Input: part model. Units: mm. Frame: model coordinates. Round coordinates to 2 decimals unless told otherwise and drop trailing zeros. Loops run counter-clockwise (first coordinate to the right, second up) from the corner with the lowest first, then second, coordinate; pieces in that order, holes last.
1) First-contact query: pin 1 (5 mm diameter, centred on x = -67, z = 0, fed in from -Y); pin 2 (1.5 mm diameter, centred on y = 1, z = 13, fed in from +X). Flat tips, straight axial feed; report the tip coordinate or a pass-through.
2) Section A-A, the plane y = 1.25. State how many separate pieces and enclosed holes the cut face has, and give its area (3 significant figures).
3) Ray query, line 1 along Z through (x, y) = (-250, 2.7); line 2 along Z through (x, y) = (-299.5, 0.8); line 3 along X through (y, z) = (1.5, -8.5). Return the intervals inside material, ascending.
4) Section B-B, the plane z = 26. Return loops of the section in (x, y).
5) Draft query along X for faces 1 (the face through (-187, 0, 0)), 2 (the face through (-294.233, 1.774, -2.999)), 3 (the face through (23.986, 1.774, 24.297)). Return one class per face: pulls with the +X half, pulls with the -X half, needs draft (parallel to the pull), parting line crosses it, or undercut.
Autodesk Inventor part; units mm, degrees
ref_plane "YZ Plane" through (0, 0, 0) normal (1, 0, 0) x (0, 1, 0)
ref_plane "XZ Plane" through (0, 0, 0) normal (0, 1, 0) x (-1, 0, 0)
ref_plane "XY Plane" through (0, 0, 0) normal (0, 0, 1) x (1, 0, 0)
sketch "Sketch1" plane through (0, 0, 0) normal (0, 1, 0) x (-1, 0, 0)
  line L0 (0, 0) -> (-16.25, 0)
  line L1 (0, 0) -> (44.75, 0)
  line L2 (300, 0) -> (330, 0)
  line L3 (330, 30) -> (-30, 30)
  line L4 (-16.25, 15.5) -> (44.75, 15.5)
  line L5 (44.75, 15.5) -> (44.75, 0)
  line L6 (44.75, -15.5) -> (-16.25, -15.5)
  line L7 (-16.25, -15.5) -> (-16.25, 0)
  line L8 (-16.25, 15.5) -> (44.75, -15.5) construction
  line L9 (44.75, 15.5) -> (-16.25, -15.5) construction
  line L10 (-20.25, 8.5) -> (48.75, 8.5) construction
  line L11 (48.75, 8.5) -> (48.75, -8.5) construction
  line L12 (48.75, -8.5) -> (-20.25, -8.5) construction
  line L13 (-20.25, -8.5) -> (-20.25, 8.5) construction
  line L14 (-20.25, 8.5) -> (48.75, -8.5) construction
  line L15 (48.75, 8.5) -> (-20.25, -8.5) construction
  line L16 (-30, 0) -> (-30, 30)
  line L17 (330, 0) -> (330, 30)
  line L18 (44.75, 0) -> (300, 0)
  line L19 (44.75, 0) -> (44.75, -15.5)
  line L20 (-16.25, 0) -> (-30, 0)
  line L21 (-16.25, 0) -> (-16.25, 15.5)
  line L22 (300, 0) -> (300, 17) construction
  line L23 (0, 0) -> (-30, 0) construction
  point P0 (14.25, 0)
  point P1 (14.25, 0)
  point P2 (289, 0)
  point P3 (67, 0)
  point P4 (250, 0)
  dimension "d0" = 300
  dimension "d5" = 61
  dimension "d6" = 31
  dimension "d7" = 69
  dimension "d8" = 17
  dimension "d9" = 16.25
  dimension "d10" = 30
  dimension "d11" = 30
  dimension "d20" = 17
  dimension "d21" = 11
  dimension "d46" = 97
  dimension "d47" = 80
extrude "Extrusion1" add sketch "Sketch1" along normal blind 3.5 contours L20 L16 L3 L17 L2 L18 L5 L4 L21
hole "Hole1" at (20.25, 0, 8.5) at (-48.75, 0, 8.5) direction (0, 1, 0) diameter 3 end through all
hole "Hole2" [suppressed]
fillet "Fillet1" radius 20 1 edges at (30, 1.75, 30)
mirror "Mirror1" about plane through (-44.75, 0, 0) normal (0, 0, -1)
hole "Hole3" at (-300, 0, 0) direction (0, 1, 0) diameter 13 end through all
hole "Hole4" at (-300, 0, 17) direction (0, 1, 0) diameter 4 end through all
pattern_linear "Rectangular Pattern1" count 5 spacing 50 along (1, 0, 0) of "Hole4"
hole "Hole5" at (-67, 0, 0) at (-250, 0, 0) direction (0, 1, 0) diameter 4.5 end through all
properties part number "segment1a" material "Plywood, Finish"
Final values:
1. pin 1: stops at y = 0
1. pin 2: stops at x = 29.87
2. separate pieces: 1
2. enclosed holes: 13
2. area: 19,300 mm2
3. line 1: z = -30 to -2.25, 2.25 to 15, 19 to 30
3. line 2: z = -30 to -6.48, 6.48 to 15.06, 18.94 to 30
3. line 3: x = -330 to -50.25, -47.25 to -44.75, 16.25 to 18.75, 21.75 to 30
4. outline: (-330, 0) - (22, 0) - (22, 3.5) - (-330, 3.5) - close
5. face 1: needs draft
5. face 2: undercut
5. face 3: pulls with the +X half
